```python
from build123d import *

# Parameters (mm, degrees)
SKETCH1_W           = 99.06
SKETCH1_H           = 203.2
BOSS_EXTRUDE1_DEPTH = 25.4
SKETCH2_R           = 49.53
SKETCH2_R_2         = 44.45
BOSS_EXTRUDE2_DEPTH = 203.2
CUT_EXTRUDE1_DEPTH  = 219.2109846
SKETCH6_W           = 38.1
SKETCH6_H           = 12.7
SKETCH6_R           = 3.175
BOSS_EXTRUDE3_DEPTH = 7.62


with BuildPart() as part:
    # Sketch1 → Boss-Extrude1 (new body)
    with BuildSketch(Plane.XY):
        Rectangle(SKETCH1_W, SKETCH1_H)
    extrude(amount=BOSS_EXTRUDE1_DEPTH)

    # Sketch2 → Boss-Extrude2 (add, through all)
    with BuildSketch(Plane(origin=(0, 101.6, 0), x_dir=(1, 0, 0), z_dir=(0, 1, 0))):
        with Locations((0, -12.7)):
            Circle(SKETCH2_R)
        with Locations((0, -12.7)):
            Circle(SKETCH2_R_2, mode=Mode.SUBTRACT)
    extrude(amount=-BOSS_EXTRUDE2_DEPTH)

    # Sketch3 → Cut-Extrude1 (cut, through all)
    with BuildSketch(Plane(origin=(0, 101.6, 0), x_dir=(1, 0, 0), z_dir=(0, 1, 0))):
        with BuildLine():
            Line((-38.01523905, 19.05), (-47.519048812, 19.05))
            ThreePointArc((-47.519048812, 19.05), (-57.15, -12.7), (-47.519048812, -44.45))
            Line((-47.519048812, -44.45), (-38.01523905, -44.45))
            ThreePointArc((-38.01523905, -44.45), (-43.988304304, -35.465104533), (-47.874115135, -25.4))
            Line((-47.874115135, -25.4), (-49.53, -25.4))
            Line((-49.53, -25.4), (-49.53, -12.7))
            Line((-49.53, -12.7), (-49.53, 0))
            Line((-49.53, 0), (-47.874115135, 0))
            ThreePointArc((-47.874115135, 0), (-43.988304304, 10.065104533), (-38.01523905, 19.05))
        make_face()
        with BuildLine():
            Line((47.519048812, 19.05), (38.01523905, 19.05))
            ThreePointArc((38.01523905, 19.05), (43.988304304, 10.065104533), (47.874115135, 0))
            Line((47.874115135, 0), (49.53, 0))
            Line((49.53, 0), (49.53, -12.7))
            Line((49.53, -12.7), (49.53, -25.4))
            Line((49.53, -25.4), (47.874115135, -25.4))
            ThreePointArc((47.874115135, -25.4), (43.988304304, -35.465104533), (38.01523905, -44.45))
            Line((38.01523905, -44.45), (47.519048812, -44.45))
            ThreePointArc((47.519048812, -44.45), (54.689286609, -29.289286609), (57.15, -12.7))
            ThreePointArc((57.15, -12.7), (54.689286609, 3.889286609), (47.519048812, 19.05))
        make_face()
        with BuildLine():
            ThreePointArc((31.108519733, 19.05), (0, 31.75), (-31.108519733, 19.05))
            Line((-31.108519733, 19.05), (31.108519733, 19.05))
        make_face()
        with BuildLine():
            ThreePointArc((38.01523905, 19.05), (0, 36.83), (-38.01523905, 19.05))
            Line((-38.01523905, 19.05), (-31.108519733, 19.05))
            ThreePointArc((-31.108519733, 19.05), (0, 31.75), (31.108519733, 19.05))
            Line((31.108519733, 19.05), (38.01523905, 19.05))
        make_face()
        with BuildLine():
            ThreePointArc((2.76e-07, 44.45), (-26.940768242, 37.701562541), (-47.519048812, 19.05))
            Line((-47.519048812, 19.05), (-38.01523905, 19.05))
            ThreePointArc((-38.01523905, 19.05), (0, 36.83), (38.01523905, 19.05))
            Line((38.01523905, 19.05), (47.519048812, 19.05))
            ThreePointArc((47.519048812, 19.05), (26.940768485, 37.701562411), (2.76e-07, 44.45))
        make_face()
        with BuildLine():
            Line((-63.5, 44.45), (-63.5, 19.05))
            Line((-63.5, 19.05), (-47.519048812, 19.05))
            ThreePointArc((-47.519048812, 19.05), (-26.940768242, 37.701562541), (2.76e-07, 44.45))
            Line((2.76e-07, 44.45), (-63.5, 44.45))
        make_face()
        with BuildLine():
            Line((63.5, 44.45), (2.76e-07, 44.45))
            ThreePointArc((2.76e-07, 44.45), (26.940768485, 37.701562411), (47.519048812, 19.05))
            Line((47.519048812, 19.05), (63.5, 19.05))
            Line((63.5, 19.05), (63.5, 44.45))
        make_face()
        with BuildLine():
            ThreePointArc((47.519048812, -44.45), (26.940768401, -63.101562456), (8.5e-08, -69.85))
            Line((8.5e-08, -69.85), (63.5, -69.85))
            Line((63.5, -69.85), (63.5, -44.45))
            Line((63.5, -44.45), (47.519048812, -44.45))
        make_face()
        with BuildLine():
            ThreePointArc((8.5e-08, -69.85), (-26.940768326, -63.101562496), (-47.519048812, -44.45))
            Line((-47.519048812, -44.45), (-63.5, -44.45))
            Line((-63.5, -44.45), (-63.5, -69.85))
            Line((-63.5, -69.85), (8.5e-08, -69.85))
        make_face()
        with BuildLine():
            Line((-38.01523905, -44.45), (-47.519048812, -44.45))
            ThreePointArc((-47.519048812, -44.45), (-26.940768326, -63.101562496), (8.5e-08, -69.85))
            ThreePointArc((8.5e-08, -69.85), (26.940768401, -63.101562456), (47.519048812, -44.45))
            Line((47.519048812, -44.45), (38.01523905, -44.45))
            ThreePointArc((38.01523905, -44.45), (0, -62.23), (-38.01523905, -44.45))
        make_face()
        with BuildLine():
            Line((-31.108519733, -44.45), (-38.01523905, -44.45))
            ThreePointArc((-38.01523905, -44.45), (0, -62.23), (38.01523905, -44.45))
            Line((38.01523905, -44.45), (31.108519733, -44.45))
            ThreePointArc((31.108519733, -44.45), (0, -57.15), (-31.108519733, -44.45))
        make_face()
        with BuildLine():
            Line((31.108519733, -44.45), (-31.108519733, -44.45))
            ThreePointArc((-31.108519733, -44.45), (0, -57.15), (31.108519733, -44.45))
        make_face()
        with BuildLine():
            ThreePointArc((-49.53, -12.7), (-49.114284188, -6.296251983), (-47.874115135, 0))
            Line((-47.874115135, 0), (-49.53, 0))
            Line((-49.53, 0), (-49.53, -12.7))
        make_face()
        with BuildLine():
            ThreePointArc((-47.874115135, -25.4), (-49.114284188, -19.103748017), (-49.53, -12.7))
            Line((-49.53, -12.7), (-49.53, -25.4))
            Line((-49.53, -25.4), (-47.874115135, -25.4))
        make_face()
        with BuildLine():
            Line((49.53, -25.4), (49.53, -12.7))
            ThreePointArc((49.53, -12.7), (49.114284188, -19.103748017), (47.874115135, -25.4))
            Line((47.874115135, -25.4), (49.53, -25.4))
        make_face()
        with BuildLine():
            Line((49.53, 0), (47.874115135, 0))
            ThreePointArc((47.874115135, 0), (49.114284188, -6.296251983), (49.53, -12.7))
            Line((49.53, -12.7), (49.53, 0))
        make_face()
    extrude(amount=-CUT_EXTRUDE1_DEPTH, mode=Mode.SUBTRACT)

    # Sketch6 → Boss-Extrude3 (add)
    # profile 1 of 2: a face of its own
    with BuildSketch(Plane.XY.offset(25.4)):
        with Locations((0, 50.8)):
            Rectangle(SKETCH6_W, SKETCH6_H)
        with Locations(Location((0, 50.8, 0), (0, 0, 180))):
            Circle(SKETCH6_R, mode=Mode.SUBTRACT)
    # profile 2 of 2: a face of its own
    with BuildSketch(Plane.XY.offset(25.4)):
        with Locations((0, -76.2)):
            Rectangle(SKETCH6_W, SKETCH6_H)
        with Locations(Location((0, -76.2, 0), (0, 0, 180))):
            Circle(SKETCH6_R, mode=Mode.SUBTRACT)
    extrude(amount=BOSS_EXTRUDE3_DEPTH)


solid = part.part
```
Input: part model. Units: mm. Frame: model coordinates. A direction names the side the tool comes from. Give positions to 0.01 mm unless a question says otherwise; leave off trailing zeros. Order: outer loops, then holes, each group sorted by start corner. A loop starts at its lowest first (then second) coordinate and runs counter-clockwise, first axis right, second up.
1. Line query: probe 1 along Y at (x, z) = (0, 28) (3 decimals); probe 2 along Y at (x, z) = (16.5, 28); probe 3 along Z at (x, y) = (41, 0). Output: solid intervals per line, ascending.
Computed:
probe 1: y = -82.55 to -79.375, -73.025 to -69.85, 44.45 to 47.625, 53.975 to 57.15
probe 2: y = -82.55 to -69.85, 44.45 to 57.15
probe 3: z = -15.09 to -4.47, 0 to 25.4, 29.87 to 40.49
2. Cut plane A-A (z = -2). Return loops of the section in (x, y).
Computed:
outline: (-47.3, -101.6) - (-41.95, -101.6) - (-41.95, 101.6) - (-47.3, 101.6) - close; (41.95, -101.6) - (47.3, -101.6) - (47.3, 101.6) - (41.95, 101.6) - close
3. Set-up query: faces 1 (the face through (-1, 1, 0)), 2 (the face through (-35, 1, 44.45)), 3 (the face through (0, -76, 25.4)), 4 (the face through (19.05, -76, 29)), 5 (the face through (-1, 1, 25.4)). Return all of +Z, -Z, +X, -X, +Y, -Y with unobstructed straight access to the full face (end or side cutting, diameter ignored); none if empty.
Computed:
face 1: +Y, -Y
face 2: +Z, +X, -X, +Y, -Y
face 3: +Z
face 4: +Z, +Y, -Y
face 5: none
4. Pin query (flat end, axial travel): pin 1 Ø8.5 at (y, z) = (51.5, 28) entering from -X; pin 2 Ø4 at (x, y) = (-3, -79.5) entering from +Z; pin 3 Ø6 at (x, z) = (9, 29.5) entering from -Y. Return the tip coordinate at first contact, or that it passes through.
Computed:
pin 1: stops at x = -48.28
pin 2: stops at z = 33.02
pin 3: stops at y = -82.55
5. Cut plane C-C (y = 67.5). Return loops of the section in (x, z).
Computed:
outline: (-42.6, 0) - (42.6, 0) arc R44.45 cw to (31.11, -19.05) - (38.02, -19.05) arc R49.53 ccw to (38.02, 44.45) - (31.11, 44.45) arc R44.45 cw to (42.6, 25.4) - (-42.6, 25.4) arc R44.45 cw to (-31.11, 44.45) - (-38.02, 44.45) arc R49.53 ccw to (-38.02, -19.05) - (-31.11, -19.05) arc R44.45 cw to start
6. Draft query along Y for faces 6 (the face through (0, 51, 25.4)), 7 (the face through (35, 1, -19.05)), 8 (the face through (0, -82.55, 29)). Return one class per face: released by +Y, released by -Y, zero draft, split by the parting line, or undercut.
Computed:
face 6: undercut
face 7: zero draft
face 8: released by -Y
7. Cut plane B-B (x = -15). Return loops of the section in (y, z), and give its area (3 significant figures).
Computed:
outline: (-101.6, 0) - (101.6, 0) - (101.6, 25.4) - (57.15, 25.4) - (57.15, 33.02) - (44.45, 33.02) - (44.45, 25.4) - (-69.85, 25.4) - (-69.85, 33.02) - (-82.55, 33.02) - (-82.55, 25.4) - (-101.6, 25.4) - close
area: 5,350 mm2
8. Cut plane D-D (z = 30). Return loops of the section in (x, y) (3 decimals).
Computed:
outline: (-46.41, -101.6) - (-40.945, -101.6) - (-40.945, 101.6) - (-46.41, 101.6) - close; (-19.05, -82.55) - (19.05, -82.55) - (19.05, -69.85) - (-19.05, -69.85) - close; (-19.05, 44.45) - (19.05, 44.45) - (19.05, 57.15) - (-19.05, 57.15) - close; (40.945, -101.6) - (46.41, -101.6) - (46.41, 101.6) - (40.945, 101.6) - close; hole circle Ø6.35 at (0, -76.2); hole circle Ø6.35 at (0, 50.8)
